Print and shaded views of the part. All mm, measured from the part's lowest x, y and z. Round coordinates to 2 decimals unless told otherwise and drop trailing zeros. Write each loop counter-clockwise with the first axis right and the second up, starting at its lowest first coordinate (ties: lowest second). Pieces come first, ordered by that corner, then holes. Notation, with made-up numbers: (12.5, -23.75) -> (47.5, -23.75) arc R34 cw to (47.5, 8.25) -> close; hole circle Ø1 at (-9, 52). An arc over 180 degrees is marked (long way). Return JSON: item names as keys, results as strings. Group by question number.
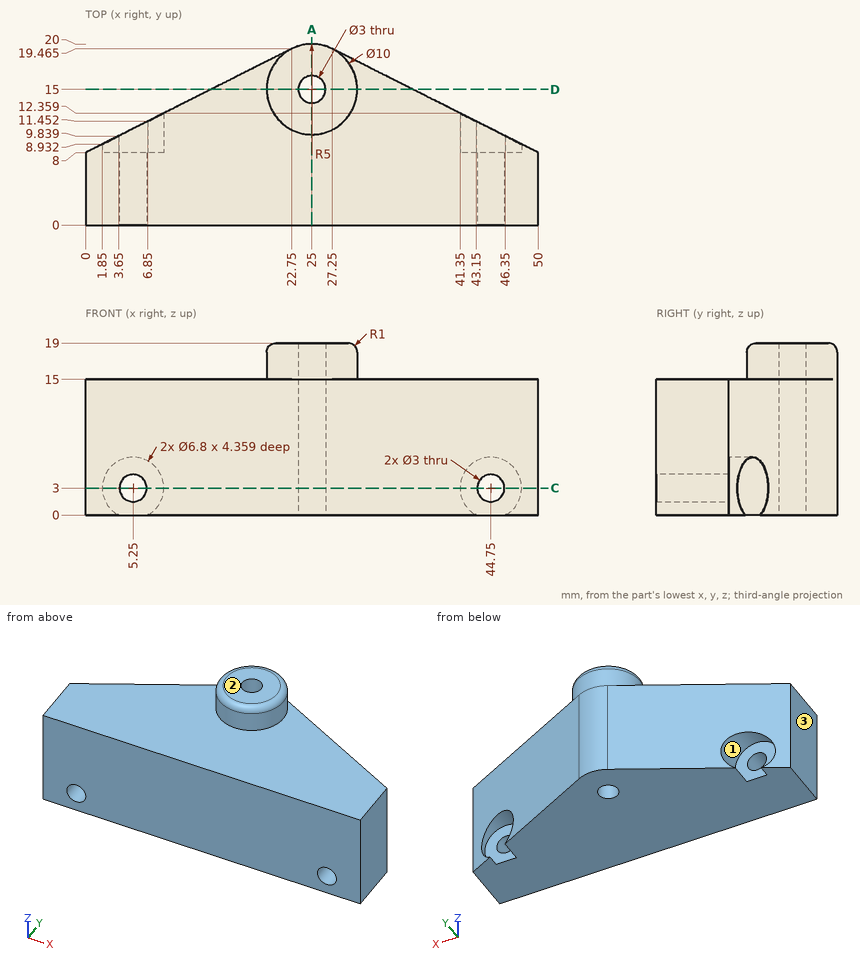
Item 1: Cut at A-A (x = 25). Write the cut outline in (y, z).
Item 2: Wall check: L1, parallel to X at y = 2.25, z = 3; L2, parallel to Z at x = 24.5, y = 5.25; L3, parallel to Z at x = 45.5, y = 5. Give the ranges that are in metal, low to high.
Item 3: Cut at C-C (z = 3). State how many separate pieces and enclosed holes the cut face has, then the cut area to 3 significant figures.
Item 4: Flat gauge pins, fed straight in: P1, Ø1.9, axis at x = 6, z = 3, coming from the +Y side; P2, Ø1.8, axis at x = 44.75, z = 3, coming from the -Y side; P3, Ø5, axis at x = 32.5, z = 9.5, coming from the +Y side; P4, Ø11, axis at x = 44.75, z = 3, coming from the +Y side. Where does each tip first touch, or does it go through?
Item 5: Cut at D-D (y = 15). Write the cut outline in (x, z), then the cut area to 3 significant figures.
Item 6: Two-plate mould, pull along X, no slides. Class the marked faces 1, 2 and 3: released by +X, released by -X, zero draft, split by the parting line, or undercut.
Checks:
{
 "1": {"outline": "(0, 0) -> (13.5, 0) -> (13.5, 19) -> (11, 19) arc R1 ccw to (10, 18) -> (10, 15) -> (0, 15) -> close; (16.5, 0) -> (20, 0) -> (20, 18) arc R1 ccw to (19, 19) -> (16.5, 19) -> close"},
 "2": {"L1": "x = 0 to 3.75, 6.75 to 43.25, 46.25 to 50", "L2": "z = 0 to 15", "L3": "z = 0 to 1.7, 4.3 to 15"},
 "3": {"separate pieces": "3", "enclosed holes": "1", "area": "623 mm2"},
 "4": {"P1": "stops at y = 8", "P2": "passes through", "P3": "stops at y = 18.08", "P4": "stops at y = 13.42"},
 "5": {"outline": "(13.89, 0) -> (23.5, 0) -> (23.5, 19) -> (21, 19) arc R1 ccw to (20, 18) -> (20, 15) -> (13.89, 15) -> close; (26.5, 0) -> (36.11, 0) -> (36.11, 15) -> (30, 15) -> (30, 18) arc R1 ccw to (29, 19) -> (26.5, 19) -> close", "area": "316 mm2"},
 "6": {"face 1": "undercut", "face 2": "zero draft", "face 3": "released by -X"}
}
